Geometry: final body of the model. Coordinates: model frame, mm. A direction names the side the tool comes from. Round coordinates to 2 decimals unless told otherwise and drop trailing zeros. Return JSON: item names as keys, results as strings.
from build123d import *

# Parameters (mm, degrees)
F0_R        = 4.998
F1_DEPTH    = 5
F2_T1_DEPTH = 65.7168298797
F4_R        = 4.99999
F6_DEPTH    = 25
F7_T1_DEPTH = 49.600858076


# Not quite as in the source:
# - a fillet or chamfer that OpenCascade refuses, or shapes differently, is made with other operations: its cross-section is extruded or revolved along the edge and cut away or added
# - a fillet or chamfer is up to 0.001 mm smaller than in the source, because OpenCascade refuses the exact size
# - a feature of the source that left no trace in its solid (it failed there, or was rolled back) is left out


with BuildPart() as f1:
    # F0 (on Top) → F1 (new body)
    with BuildSketch(Plane.XY):
        with BuildLine():
            Line((-18.0062504657, -20), (21.9937495343, -20))
            Line((21.9937495343, -20), (21.9937495343, 20))
            Line((21.9937495343, 20), (-8.0062504657, 20))
            ThreePointArc((-8.0062504657, 20), (-15.0773182775, 17.0710678119), (-18.0062504657, 10))
            Line((-18.0062504657, 10), (-18.0062504657, -20))
        make_face()
        Circle(F0_R, mode=Mode.SUBTRACT)
    extrude(amount=F1_DEPTH)

    # F2: chamfer of 5 on 1 edges, made by hand

    # F2_s2 → F2_t1 (cut)
    with BuildSketch(Plane.YZ.offset(-30.8646654055)):
        Polygon((-20, 0), (-15, 5), (-20, 5), align=None)
    extrude(amount=F2_T1_DEPTH, mode=Mode.SUBTRACT)

    # F4 (radius 5 in the source; OpenCascade refuses exactly that, so slightly less here)
    f4_edges = [f1.edges().sort_by_distance(p)[0] for p in [
        (21.99375, 2.5, 5),
        (-18.00625, -2.5, 5),
        (-15.077318, 17.071068, 5),
        (6.99375, 20, 5),
    ]]
    fillet(f4_edges, radius=F4_R)

    # F5 (on face) → F6 (join)
    with BuildSketch(Plane(origin=(0, -10, 10), x_dir=(1, 0, 0), z_dir=(0, -0.7071067812, 0.7071067812))):
        with BuildLine():
            Line((-16.3453794084, -11.8680624291), (7.5386487879, -11.8680624291))
            Line((7.5386487879, -11.8680624291), (7.5386487879, -7.0710678119))
            Line((7.5386487879, -7.0710678119), (-13.0062604657, -7.0710678119))
            add(Edge.make_bspline(
                [(-16.3453794084, -8.8790074441), (-14.9205436029, -7.0710678119), (-13.0062604657, -7.0710678119)],
                knots=[2.4075114321, 2.4075114321, 2.4075114321, 3.1415926536, 3.1415926536, 3.1415926536], degree=2, weights=[0.8541785937, 0.8631220304, 1]))
            Line((-16.3453794084, -8.8790074441), (-16.3453794084, -11.8680624291))
        make_face()
    extrude(amount=F6_DEPTH)

    # F7: chamfer of 5 on 1 edges, made by hand

    # F7_s2 → F7_t1 (cut)
    with BuildSketch(Plane.YZ.offset(-29.2037943483)):
        Polygon((-32.5341230469, 15.7501482005), (-32.5341230469, 22.8212160124), (-36.0696569528, 19.2856821065), align=None)
    extrude(amount=F7_T1_DEPTH, mode=Mode.SUBTRACT)


solid = f1.part
Q1. Pull-direction query (Y, two-part tool) for faces 5 (the flat face through (6, 0, 0)), 6 (the cylindrical face through (7, 19, 3)), 7 (the flat face through (-4.571, -25.364, 8.58)), 8 (the cylindrical face through (3, 4, 2)); classes: pulls with the +Y half, pulls with the -Y half, needs draft (parallel to the pull), parting line crosses it, or undercut.
Determined:
{"face 5": "needs draft", "face 6": "pulls with the +Y half", "face 7": "pulls with the -Y half", "face 8": "undercut"}
Q2. Material intervals for L1, parallel to Z at x = 11.5, y = -8; L2, parallel to Y at x = 0, z = 1.1; L3, parallel to X at y = -28, z = 15.25, sorted ascending.
Determined:
{"L1": "z = 0 to 5", "L2": "y = -18.9 to -5, 5 to 19.88", "L3": "x = -16.35 to 7.54"}
Q3. Reachability of faces 1 (the flat face through (-5, -32.534, 19)), 2 (the cylindrical face through (-16.58, -5.21, 3.496)), 3 (the flat face through (7.539, -25, 12)), 4 (the flat face through (5, -3, 5)) from +Z, -Z, +X, -X, +Y, -Y: full face, straight path, thin tool, end or side. Return the list, or none.
Determined:
{"face 1": "+Z, -Z, +X, -X, -Y", "face 2": "+Z, -X, +Y", "face 3": "+Z, +X, -Y", "face 4": "+Z, +X, -X, +Y"}
Q4. Pin query (flat end, axial travel): pin 1 (4 mm diameter, centred on x = 7.5, z = 10.5, fed in from -Y); pin 2 (8 mm diameter, centred on y = -5, z = 6.5, fed in from -X); pin 3 (10 mm diameter, centred on y = -23, z = 19.5, fed in from -X). Return the tip coordinate at first contact, or that it passes through.
Determined:
{"pin 1": "stops at y = -29.28", "pin 2": "stops at x = -17.34", "pin 3": "stops at x = -14.67"}
